```python
from build123d import *

# Parameters (mm, degrees)
EXTRUDE_1_DEPTH      = 61.6
SHELL_1_T            = -2
CUT_EXTRUDE_8_DEPTH  = 3.5
CUT_EXTRUDE_9_REACH  = 80.817
CUT_EXTRUDE_10_REACH = 80.817
CUT_EXTRUDE_11_REACH = 86.711
CUT_EXTRUDE_12_REACH = 86.711
CUT_EXTRUDE_13_DEPTH = 3.5
FILLET_1_R           = 3
FILLET_2_R           = 3


with BuildPart() as part:
    # ｽｹｯﾁ2 → ﾎﾞｽ - 押し出し1 (new body)
    with BuildSketch(Plane(origin=(0, 0, 0), x_dir=(0, 0, -1), z_dir=(1, 0, 0))):
        with BuildLine():
            Line((7.125790142, 45.158487371), (-0.55, 45.158487371))
            Line((-0.55, 45.158487371), (-0.55, -9.641512629))
            Line((-0.55, -9.641512629), (7.125790142, -9.641512629))
            ThreePointArc((7.125790142, -9.641512629), (15.840322505, -6.031835134), (19.45, 2.682697229))
            Line((19.45, 2.682697229), (19.45, 32.834277513))
            ThreePointArc((19.45, 32.834277513), (15.840322505, 41.548809876), (7.125790142, 45.158487371))
        make_face()
    extrude(amount=EXTRUDE_1_DEPTH)

    # ｼｪﾙ1
    shell_1_openings = [part.faces().sort_by_distance(p)[0] for p in [
        (30.8, 17.758487371, 0.55),
    ]]
    offset(amount=SHELL_1_T, openings=shell_1_openings, kind=Kind.INTERSECTION)

    # ｽｹｯﾁ11 → ｶｯﾄ - 押し出し8 (cut, symmetric)
    with BuildSketch(Plane(origin=(0, 17.758487371, 0), x_dir=(1, 0, 0), z_dir=(0, 1, 0))):
        Polygon((2.16, 2.171540251), (1.251335836, 1.262876087), (1.251335836, 0.566601917), (2.16, 0.566601917), align=None)
        Polygon((59.44, 2.171540251), (59.44, 0.566601917), (60.348664164, 0.566601917), (60.348664164, 1.262876087), align=None)
    extrude(amount=CUT_EXTRUDE_8_DEPTH, both=True, mode=Mode.SUBTRACT)

    # ｽｹｯﾁ12 → ｶｯﾄ - 押し出し9 (cut, up to next)
    with BuildSketch(Plane(origin=(61.6, 0, 0), x_dir=(0, 0, -1), z_dir=(1, 0, 0)), mode=Mode.PRIVATE) as cut_extrude_9_sk1:
        with BuildLine():
            Line((-0.55, 41.757639853), (-0.55, 29.95933489))
            ThreePointArc((-0.55, 29.95933489), (2.45, 35.858487371), (-0.55, 41.757639853))
        make_face()
    cut_extrude_9_tool1 = extrude(cut_extrude_9_sk1.sketch, amount=-CUT_EXTRUDE_9_REACH, mode=Mode.PRIVATE) & part.part
    # ｽｹｯﾁ12 → ｶｯﾄ - 押し出し9 (cut, up to next)
    with BuildSketch(Plane(origin=(61.6, 0, 0), x_dir=(0, 0, -1), z_dir=(1, 0, 0)), mode=Mode.PRIVATE) as cut_extrude_9_sk2:
        with BuildLine():
            Line((-0.55, 5.557639853), (-0.55, -6.24066511))
            ThreePointArc((-0.55, -6.24066511), (2.45, -0.341512629), (-0.55, 5.557639853))
        make_face()
    cut_extrude_9_tool2 = extrude(cut_extrude_9_sk2.sketch, amount=-CUT_EXTRUDE_9_REACH, mode=Mode.PRIVATE) & part.part
    add(cut_extrude_9_tool1.solids().sort_by_distance((61.6, 35.858487, -0.674015))[0], mode=Mode.SUBTRACT)
    add(cut_extrude_9_tool2.solids().sort_by_distance((61.6, -0.341513, -0.674015))[0], mode=Mode.SUBTRACT)

    # ｽｹｯﾁ13 → ｶｯﾄ - 押し出し10 (cut, up to next)
    with BuildSketch(Plane.ZY, mode=Mode.PRIVATE) as cut_extrude_10_sk1:
        with BuildLine():
            Line((0.55, 29.95933489), (0.55, 41.757639853))
            ThreePointArc((0.55, 41.757639853), (-2.45, 35.858487371), (0.55, 29.95933489))
        make_face()
    cut_extrude_10_tool1 = extrude(cut_extrude_10_sk1.sketch, amount=-CUT_EXTRUDE_10_REACH, mode=Mode.PRIVATE) & part.part
    # ｽｹｯﾁ13 → ｶｯﾄ - 押し出し10 (cut, up to next)
    with BuildSketch(Plane.ZY, mode=Mode.PRIVATE) as cut_extrude_10_sk2:
        with BuildLine():
            Line((0.55, -6.24066511), (0.55, 5.557639853))
            ThreePointArc((0.55, 5.557639853), (-2.45, -0.341512629), (0.55, -6.24066511))
        make_face()
    cut_extrude_10_tool2 = extrude(cut_extrude_10_sk2.sketch, amount=-CUT_EXTRUDE_10_REACH, mode=Mode.PRIVATE) & part.part
    add(cut_extrude_10_tool1.solids().sort_by_distance((0, 35.858487, -0.674015))[0], mode=Mode.SUBTRACT)
    add(cut_extrude_10_tool2.solids().sort_by_distance((0, -0.341513, -0.674015))[0], mode=Mode.SUBTRACT)

    # ｽｹｯﾁ14 → ｶｯﾄ - 押し出し11 (cut, up to next)
    with BuildSketch(Plane.XZ.offset(9.641512629), mode=Mode.PRIVATE) as cut_extrude_11_sk1:
        with BuildLine():
            Line((5.300847518, 0.55), (17.099152482, 0.55))
            ThreePointArc((17.099152482, 0.55), (11.2, -2.45), (5.300847518, 0.55))
        make_face()
    cut_extrude_11_tool1 = extrude(cut_extrude_11_sk1.sketch, amount=-CUT_EXTRUDE_11_REACH, mode=Mode.PRIVATE) & part.part
    # ｽｹｯﾁ14 → ｶｯﾄ - 押し出し11 (cut, up to next)
    with BuildSketch(Plane.XZ.offset(9.641512629), mode=Mode.PRIVATE) as cut_extrude_11_sk2:
        with BuildLine():
            Line((44.500847518, 0.55), (56.299152482, 0.55))
            ThreePointArc((56.299152482, 0.55), (50.4, -2.45), (44.500847518, 0.55))
        make_face()
    cut_extrude_11_tool2 = extrude(cut_extrude_11_sk2.sketch, amount=-CUT_EXTRUDE_11_REACH, mode=Mode.PRIVATE) & part.part
    add(cut_extrude_11_tool1.solids().sort_by_distance((11.2, -9.641513, -0.674015))[0], mode=Mode.SUBTRACT)
    add(cut_extrude_11_tool2.solids().sort_by_distance((50.4, -9.641513, -0.674015))[0], mode=Mode.SUBTRACT)

    # ｽｹｯﾁ15 → ｶｯﾄ - 押し出し12 (cut, up to next)
    with BuildSketch(Plane(origin=(0, 45.158487371, 0), x_dir=(1, 0, 0), z_dir=(0, 1, 0)), mode=Mode.PRIVATE) as cut_extrude_12_sk1:
        with BuildLine():
            Line((44.500847518, -0.55), (56.299152482, -0.55))
            ThreePointArc((56.299152482, -0.55), (50.4, 2.45), (44.500847518, -0.55))
        make_face()
    cut_extrude_12_tool1 = extrude(cut_extrude_12_sk1.sketch, amount=-CUT_EXTRUDE_12_REACH, mode=Mode.PRIVATE) & part.part
    # ｽｹｯﾁ15 → ｶｯﾄ - 押し出し12 (cut, up to next)
    with BuildSketch(Plane(origin=(0, 45.158487371, 0), x_dir=(1, 0, 0), z_dir=(0, 1, 0)), mode=Mode.PRIVATE) as cut_extrude_12_sk2:
        with BuildLine():
            Line((5.300847518, -0.55), (17.099152482, -0.55))
            ThreePointArc((17.099152482, -0.55), (11.2, 2.45), (5.300847518, -0.55))
        make_face()
    cut_extrude_12_tool2 = extrude(cut_extrude_12_sk2.sketch, amount=-CUT_EXTRUDE_12_REACH, mode=Mode.PRIVATE) & part.part
    add(cut_extrude_12_tool1.solids().sort_by_distance((50.4, 45.158487, -0.674015))[0], mode=Mode.SUBTRACT)
    add(cut_extrude_12_tool2.solids().sort_by_distance((11.2, 45.158487, -0.674015))[0], mode=Mode.SUBTRACT)

    # ｽｹｯﾁ16 → ｶｯﾄ - 押し出し13 (cut, symmetric)
    with BuildSketch(Plane(origin=(30.8, 0, 0), x_dir=(0, 0, -1), z_dir=(1, 0, 0))):
        Polygon((2.051421356, 43.058487371), (0.651335836, 43.058487371), (0.651335836, 43.847151535), (1.262757192, 43.847151535), align=None)
        Polygon((1.262757192, -8.330176793), (2.051421356, -7.541512629), (0.651335836, -7.541512629), (0.651335836, -8.330176793), align=None)
    extrude(amount=CUT_EXTRUDE_13_DEPTH, both=True, mode=Mode.SUBTRACT)

    # ﾌｨﾚｯﾄ1
    fillet_1_edges = [part.edges().sort_by_distance(p)[0] for p in [
        (61.6, -6.031835134, -15.840322505),
        (61.6, 17.758487371, -19.45),
        (61.6, 41.548809876, -15.840322505),
        (61.6, 45.158487371, -3.287895071),
        (61.6, -9.641512629, -3.287895071),
    ]]
    fillet(fillet_1_edges, radius=FILLET_1_R)

    # ﾌｨﾚｯﾄ2
    fillet_2_edges = [part.edges().sort_by_distance(p)[0] for p in [
        (0, 45.158487371, -3.287895071),
        (0, 41.548809876, -15.840322505),
        (0, 17.758487371, -19.45),
        (0, -6.031835134, -15.840322505),
        (0, -9.641512629, -3.287895071),
    ]]
    fillet(fillet_2_edges, radius=FILLET_2_R)


solid = part.part
```
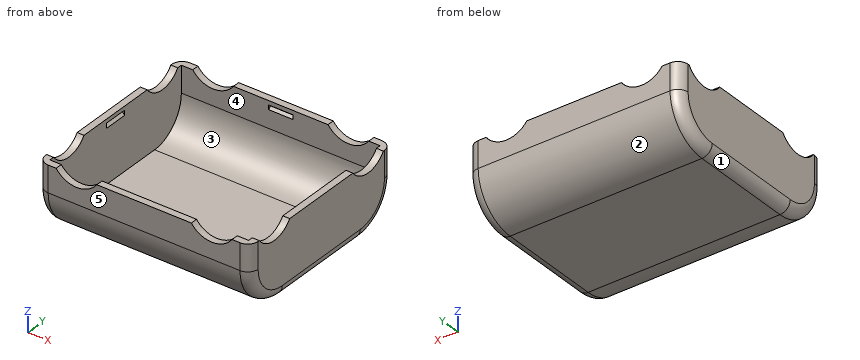
Verification items for the finished model (mm, model axes). Face numbers are marked on the shaded views. A direction names the side the tool comes from. Round coordinates to 2 decimals unless told otherwise and drop trailing zeros. Loops run counter-clockwise (first coordinate to the right, second up) from the corner with the lowest first, then second, coordinate; pieces in that order, holes last. Notation, with made-up numbers: (58.5, -12.75) -> (82.5, -12.75) arc R23 ccw to (82.5, 3.25) -> close; hole circle Ø2 at (-33, 55.5). An arc over 180 degrees is marked (long way). Answer as a JSON object with one key per item and string values.
Q1. Draft check along Y on the marked faces 1, 2 and 3. Enter one of: pulls with the +Y half, pulls with the -Y half, needs draft (parallel to the pull), parting line crosses it, or undercut.
Data:
{"face 1": "needs draft", "face 2": "pulls with the +Y half", "face 3": "undercut"}
Q2. Access from +Z, -Z, +X, -X, +Y, -Y to the whole of each face (thin tool, end or side, straight path). Record for the marked faces 4 and 5.
Data:
{"face 4": "+Z", "face 5": "+Z, -Z, +X, -X, -Y"}
Q3. Section check A-A (z = -4.5). Record the boundary of the cut face in (x, y).
Data:
{"outline": "(0, -6.64) arc R3 ccw to (3, -9.64) -> (58.6, -9.64) arc R3 ccw to (61.6, -6.64) -> (61.6, 42.16) arc R3 ccw to (58.6, 45.16) -> (3, 45.16) arc R3 ccw to (0, 42.16) -> close; hole (2, -7.64) -> (59.6, -7.64) -> (59.6, 43.16) -> (2, 43.16) -> close"}
Q4. Section check D-D (y = 8). Record the boundary of the cut face in (x, z), then the cut area to 3 significant figures.
Data:
{"outline": "(0, -16.45) arc R3 ccw to (3, -19.45) -> (58.6, -19.45) arc R3 ccw to (61.6, -16.45) -> (61.6, 0.55) -> (59.6, 0.55) -> (59.6, -17.45) -> (2, -17.45) -> (2, 0.55) -> (0, 0.55) -> close", "area": "191 mm2"}
Q5. Section check C-C (y = 15). Record the boundary of the cut face in (x, z), then the cut area to 3 significant figures.
Data:
{"outline": "(0, -16.45) arc R3 ccw to (3, -19.45) -> (58.6, -19.45) arc R3 ccw to (61.6, -16.45) -> (61.6, 0.55) -> (59.6, 0.55) -> (59.6, -0.57) -> (60.35, -0.57) -> (60.35, -1.26) -> (59.6, -2.01) -> (59.6, -17.45) -> (2, -17.45) -> (2, -2.01) -> (1.25, -1.26) -> (1.25, -0.57) -> (2, -0.57) -> (2, 0.55) -> (0, 0.55) -> close", "area": "190 mm2"}
Q6. Scan lines: line 1 (Y direction, x = 28.5, z = -7); line 2 (X direction, y = 37.5, z = -8); line 3 (Z direction, x = 46.5, y = 19.5). Record each from-to range of solid material in increasing order. Write a range as from..to.
Data:
{"line 1": "y = -9.64..-7.64, 43.16..45.16", "line 2": "x = 0..2, 59.6..61.6", "line 3": "z = -19.45..-17.45"}
Q7. Section check B-B (x = 30.5). Record the boundary of the cut face in (y, z).
Data:
{"outline": "(-9.64, -7.13) arc R12.32 ccw to (2.68, -19.45) -> (32.83, -19.45) arc R12.32 ccw to (45.16, -7.13) -> (45.16, 0.55) -> (43.16, 0.55) -> (43.16, -0.65) -> (43.85, -0.65) -> (43.85, -1.26) -> (43.16, -1.95) -> (43.16, -7.13) arc R10.32 cw to (32.83, -17.45) -> (2.68, -17.45) arc R10.32 cw to (-7.64, -7.13) -> (-7.64, -1.95) -> (-8.33, -1.26) -> (-8.33, -0.65) -> (-7.64, -0.65) -> (-7.64, 0.55) -> (-9.64, 0.55) -> close"}
Q8. Go/stop test with flat-tipped pins: P1, Ø1.5, axis at x = 43.5, z = -12.5, coming from the -Y side; P2, Ø0.6, axis at x = 1.5, y = 16.5, coming from the -Z side; P3, Ø24, axis at x = 20, y = 11, coming from the +Z side. Record where each tip stops, or that it passes through.
Data:
{"P1": "stops at y = -8.74", "P2": "stops at z = -19.2", "P3": "stops at z = -16.77"}
